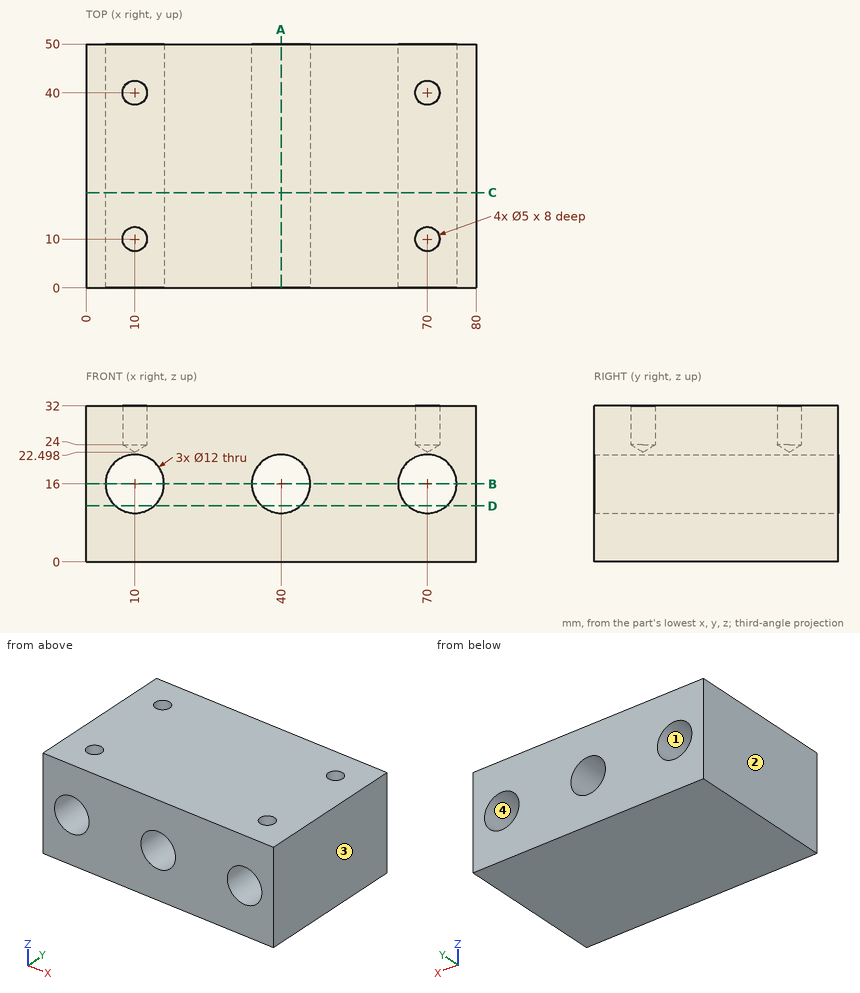
Drawing for the job (mm, zero at the part's lowest x, y, z). Give positions to 0.01 mm unless a question says otherwise; leave off trailing zeros. Order: outer loops, then holes, each group sorted by start corner. A loop starts at its lowest first (then second) coordinate and runs counter-clockwise, first axis right, second up. Notation, with made-up numbers: M 74,52.25 L 98,52.25 A17 ccw 98,70.25 Z; hole C -33.75,13 d7. An arc over 180 degrees is marked long. Write item = value, one per line. Start each with the question number.
(1) Slice it at A-A on x = 40. Write the cut outline in (y, z), plus the area to 3 significant figures.
(2) Two-plate mould, pull along X, no slides. Class the marked faces 1, 2, 3 and 4: released by +X, released by -X, zero draft, split by the parting line, or undercut.
(3) Probe L1, parallel to Y at x = 70, z = 30; L2, parallel to X at y = 40, z = 29.25; L3, parallel to Z at x = 40, y = 11. List the from-to ranges inside material, lowest first. Write a range as [from, to].
(4) Slice it at B-B on z = 16. Write the cut outline in (x, y).
(5) Pin check, flat tips, straight feed: pin 1 Ø4 at (x, y) = (70, 40) entering from +Z; pin 2 Ø9.5 at (x, z) = (70, 16) entering from +Y; pin 3 Ø3 at (x, y) = (10, 10) entering from +Z. Stop position of each tip, or through.
(6) Slice it at D-D on z = 11.5. Write the cut outline in (x, y).
(7) Slice it at C-C on y = 19.5. Write the cut outline in (x, z), plus the area to 3 significant figures.
Responses:
q1.outline = M 0,0 L 50,0 L 50,10 L 0,10 Z; M 0,22 L 50,22 L 50,32 L 0,32 Z
q1.area = 1,000 mm2
q2.face_1 = undercut
q2.face_2 = released by -X
q2.face_3 = released by +X
q2.face_4 = undercut
q3.L1 = [0, 7.5], [12.5, 37.5], [42.5, 50]
q3.L2 = [0, 7.5], [12.5, 67.5], [72.5, 80]
q3.L3 = [0, 10], [22, 32]
q4.outline = M 0,0 L 4,0 L 4,50 L 0,50 Z; M 16,0 L 34,0 L 34,50 L 16,50 Z; M 46,0 L 64,0 L 64,50 L 46,50 Z; M 76,0 L 80,0 L 80,50 L 76,50 Z
q5.pin_1 = 23.7
q5.pin_2 = through
q5.pin_3 = 23.4
q6.outline = M 0,0 L 6.03,0 L 6.03,50 L 0,50 Z; M 13.97,0 L 36.03,0 L 36.03,50 L 13.97,50 Z; M 43.97,0 L 66.03,0 L 66.03,50 L 43.97,50 Z; M 73.97,0 L 80,0 L 80,50 L 73.97,50 Z
q7.outline = M 0,0 L 80,0 L 80,32 L 0,32 Z; hole C 10,16 d12; hole C 40,16 d12; hole C 70,16 d12
q7.area = 2,220 mm2
